```python
from build123d import *

# Parameters (mm, degrees)
SKETCH1_R           = 37.5
BOSS_EXTRUDE1_DEPTH = 13
SKETCH4_R           = 27.5
CUT_EXTRUDE1_DEPTH  = 2
SKETCH5_R           = 16
BOSS_EXTRUDE2_DEPTH = 2
SKETCH6_R           = 7
CUT_EXTRUDE2_DEPTH  = 27
FILLET1_R           = 1


with BuildPart() as part:
    # Sketch1 → Boss-Extrude1 (new body, symmetric)
    with BuildSketch(Plane.XY):
        Circle(SKETCH1_R)
    extrude(amount=BOSS_EXTRUDE1_DEPTH, both=True)

    # Sketch4 → Cut-Extrude1 (cut)
    with BuildSketch(Plane(origin=(0, 0, -13), x_dir=(-1, 0, 0), z_dir=(0, 0, -1))):
        Circle(SKETCH4_R)
    cut_extrude1 = extrude(amount=-CUT_EXTRUDE1_DEPTH, mode=Mode.SUBTRACT)

    # Mirror1: Cut-Extrude1 across plane
    add(cut_extrude1.mirror(Plane.XY), mode=Mode.SUBTRACT)

    # Sketch5 → Boss-Extrude2 (add)
    with BuildSketch(Plane(origin=(0, 0, -11), x_dir=(-1, 0, 0), z_dir=(0, 0, -1))):
        Circle(SKETCH5_R)
    boss_extrude2 = extrude(amount=BOSS_EXTRUDE2_DEPTH)

    # Mirror2: Boss-Extrude2 across plane
    add(boss_extrude2.mirror(Plane.XY))

    # Sketch6 → Cut-Extrude2 (cut, through all)
    with BuildSketch(Plane(origin=(0, 0, -13), x_dir=(-1, 0, 0), z_dir=(0, 0, -1))):
        Circle(SKETCH6_R)
    extrude(amount=-CUT_EXTRUDE2_DEPTH, mode=Mode.SUBTRACT)

    # Fillet1
    fillet1_edges = [part.edges().sort_by_distance(p)[0] for p in [
        (16, 0, -13),
        (-37.5, 0, 13),
        (-37.5, 0, -13),
        (27.5, 0, -13),
    ]]
    fillet(fillet1_edges, radius=FILLET1_R)


solid = part.part
```
Geometry: final body of the model. Coordinates: model frame, mm. A direction names the side the tool comes from. Give positions to 0.01 mm unless a question says otherwise; leave off trailing zeros. Loops run counter-clockwise (first coordinate to the right, second up) from the corner with the lowest first, then second, coordinate; pieces in that order, holes last. Notation, with made-up numbers: (80.5, 74.25) -> (104.5, 74.25) arc R26 ccw to (104.5, 107.25) -> close; hole circle Ø8 at (-23, 62). An arc over 180 degrees is marked (long way). Use CSV: the item, a comma, the result in double quotes.
(1) Pull-direction query (X, two-part tool) for faces 1 (the face through (-12, -12, 11)), 2 (the face through (-3.1, -6.5, -13)), 3 (the face through (-4.88, 37.18, 0.17)); classes: released by +X, released by -X, zero draft, split by the parting line, or undercut.
From the geometry:
face 1,"undercut"
face 2,"zero draft"
face 3,"split by the parting line"
(2) Ray query, line 1 along Y through (x, z) = (0, -11.7); line 2 along Z through (x, y) = (9.5, 17); line 3 along Y through (x, z) = (0, 0.75). Return the intervals inside material, ascending. Write a range as [from, to].
From the geometry:
line 1,"[-37.5, -27.5], [-16, -7], [7, 16], [27.5, 37.5]"
line 2,"[-11, 11]"
line 3,"[-37.5, -7], [7, 37.5]"
(3) Access query for faces 4 (the face through (-6.466, -2.681, -0.182)), 5 (the face through (3.47, -15.62, 11.99)), 6 (the face through (3.47, -15.62, -11.49)). Directions: +Z, -Z, +X, -X, +Y, -Y. A direction counts if a zero-diameter tool reaches every point of the face in a straight line with its end or side. Return the directions, or none.
From the geometry:
face 4,"+Z, -Z"
face 5,"+Z"
face 6,"-Z"
(4) First-contact query: P1, Ø1.5, axis at y = -27, z = 5, coming from the +X side; P2, Ø1, axis at x = 5, z = -9.5, coming from the +Y side; P3, Ø10, axis at y = 6.5, z = 4, coming from the -X side; P4, Ø12.5, axis at x = 0, y = 0, coming from the -Z side. Flat tips, straight axial feed; report the tip coordinate or a pass-through.
From the geometry:
P1,"x = 26.78"
P2,"y = 37.23"
P3,"x = -37.47"
P4,"through"
(5) Cut plane C-C (z = 8.5). Output: boundary loops of the cut face in (x, y), plus the area to 3 significant figures.
From the geometry:
outline,"circle Ø75 at (0, 0); hole circle Ø14 at (0, 0)"
area,"4,260 mm^2"
